For this review, take the finished solid that the model builds, in its own axes (mm). Face numbers are marked on the shaded views. A direction names the side the tool comes from. Give positions to 0.01 mm unless a question says otherwise; leave off trailing zeros. Order: outer loops, then holes, each group sorted by start corner. A loop starts at its lowest first (then second) coordinate and runs counter-clockwise, first axis right, second up. Notation, with made-up numbers: (8.5, 58) - (44.5, 58) arc R19 ccw to (44.5, 93) - close; hole circle Ø9 at (62.5, 10.25). An arc over 180 degrees is marked (long way). Use a Markdown table: item, result. Add a question column.
1) Machinability: for the marked faces 4, 5 and 6, which of the approach directions +Z, -Z, +X, -X, +Y, -Y give a long, thin tool a straight path to every point of the face, cutting with its end or side? Answer none if there is none.
2) Wall thickness on L1, parallel to X at y = 5, z = -29.5; L2, parallel to Z at x = 32, y = 4.75; L3, parallel to Y at x = 35, z = -43: over which ranges is each line inside the solid? List them lowest first.
3) We need section A-A on z = -21.5. Write out the cut boundary in (x, y).
4) We need section D-D on z = -36. Write out the cut boundary in (x, y), then the cut area to 3 significant figures.
5) Clearance check with flat-ended pins moving along their axes: P1, Ø5, axis at x = 15.5, y = 3, coming from the -Z side; P2, Ø1.5, axis at x = 16.5, y = -1, coming from the -Z side; P3, Ø8, axis at x = 19, y = 4, coming from the +Z side; P4, Ø4.5, axis at x = 42.5, y = 5, coming from the +Z side. State where each tip first meets the part, or that it passes through.
6) Mouldability with a two-part tool opening along X and no side actions: class the marked faces 1, 2 and 3 as released by +X, released by -X, zero draft, split by the parting line, or undercut.
7) We need section B-B on y = 1.75. Write out the cut boundary in (x, z).
8) We need section C-C on x = 29. Write out the cut boundary in (y, z).
```python
from build123d import *

# Parameters (mm, degrees)
BOSS_EXTRUDE1_DEPTH = 10
SKETCH2_R           = 2.5
BOSS_EXTRUDE2_DEPTH = 5


with BuildPart() as part:
    # Sketch1 → Boss-Extrude1 (new body)
    with BuildSketch(Plane(origin=(0, 0, 0), x_dir=(1, 0, 0), z_dir=(0, 1, 0))):
        Polygon((21.277713785, 48.057856326), (33.277713785, 48.057856326), (33.277713785, 44.431129223), (45.277713785, 43.046501314), (45.277713785, 19.507826857), (41.027713785, 19.507826857), (41.027713785, 31.507826857), (31.027713785, 31.507826857), (29.527713785, 2.057856326), (25.027713785, 2.057856326), (23.527713785, 31.507826857), (13.527713785, 31.507826857), (13.527713785, 19.507826857), (9.277713785, 19.507826857), (9.277713785, 43.046501314), (21.277713785, 44.431129223), align=None)
    extrude(amount=BOSS_EXTRUDE1_DEPTH)

    # Sketch2 → Boss-Extrude2 (add)
    with BuildSketch(Plane(origin=(0, 0, 0), x_dir=(-1, 0, 0), z_dir=(0, -1, 0))):
        with Locations((-27.277713785, 30.711934537)):
            Circle(SKETCH2_R)
    extrude(amount=BOSS_EXTRUDE2_DEPTH)


solid = part.part
```
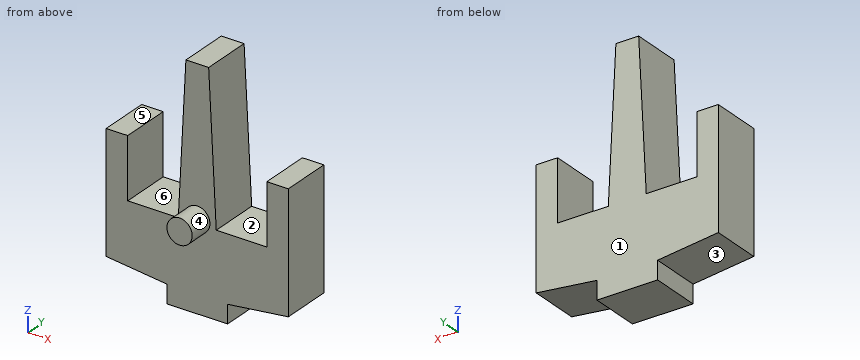
Checked values:
| question | item | result |
|---|---|---|
| 1 | face 4 | -Y |
| 1 | face 5 | +Z, -X, +Y, -Y |
| 1 | face 6 | +Z, +Y, -Y |
| 2 | L1 | 9.28 to 13.53, 23.63 to 30.93, 41.03 to 45.28 |
| 2 | L2 | -48.06 to -31.51 |
| 2 | L3 | 0 to 10 |
| 3 | outline | (9.28, 0) - (13.53, 0) - (13.53, 10) - (9.28, 10) - close; (24.04, 0) - (30.52, 0) - (30.52, 10) - (24.04, 10) - close; (41.03, 0) - (45.28, 0) - (45.28, 10) - (41.03, 10) - close |
| 4 | outline | (9.28, 0) - (45.28, 0) - (45.28, 10) - (9.28, 10) - close |
| 4 | area | 360 mm² |
| 5 | P1 | z = -44.05 |
| 5 | P2 | through |
| 5 | P3 | z = -31.51 |
| 5 | P4 | z = -19.51 |
| 6 | face 1 | zero draft |
| 6 | face 2 | undercut |
| 6 | face 3 | released by -X |
| 7 | outline | (9.28, -43.05) - (21.28, -44.43) - (21.28, -48.06) - (33.28, -48.06) - (33.28, -44.43) - (45.28, -43.05) - (45.28, -19.51) - (41.03, -19.51) - (41.03, -31.51) - (31.03, -31.51) - (29.53, -2.06) - (25.03, -2.06) - (23.53, -31.51) - (13.53, -31.51) - (13.53, -19.51) - (9.28, -19.51) - close |
| 8 | outline | (-5, -32.52) - (0, -32.52) - (0, -48.06) - (10, -48.06) - (10, -2.06) - (0, -2.06) - (0, -28.9) - (-5, -28.9) - close |
